from build123d import *

# Parameters (mm, degrees)
SKETCH1_W                                           = 52
SKETCH1_H                                           = 100
BOSS_EXTRUDE1_DEPTH                                 = 5
BOSS_EXTRUDE3_DEPTH                                 = 2.5
SKETCH7_R                                           = 2.25
BOSS_EXTRUDE4_DEPTH                                 = 2.5
FILLET2_R                                           = 0.25
SKETCH9_W                                           = 52
SKETCH9_H                                           = 2
BOSS_EXTRUDE5_DEPTH                                 = 50
BOSS_EXTRUDE7_DEPTH                                 = 52
CUT_EXTRUDE3_DEPTH                                  = 52
CUT_EXTRUDE4_DEPTH                                  = 2.5
BOSS_EXTRUDE8_DEPTH                                 = 52
BOSS_EXTRUDE9_DEPTH                                 = 4
LPATTERN1_COUNT                                     = 2
LPATTERN1_PITCH                                     = 48
SKETCH18_R                                          = 11.5
CUT_EXTRUDE5_DEPTH                                  = 2
CSK_FOR_M3_COUNTERSUNK_FLAT_HEAD_SCREW1_D           = 3.4
CSK_FOR_M3_COUNTERSUNK_FLAT_HEAD_SCREW1_DEPTH       = 5
CSK_FOR_M3_COUNTERSUNK_FLAT_HEAD_SCREW1_CSINK_D     = 6.3
CSK_FOR_M3_COUNTERSUNK_FLAT_HEAD_SCREW1_CSINK_ANGLE = 90
CSK_FOR_M3_COUNTERSUNK_FLAT_HEAD_SCREW1_TIP         = 1.021463052
BOSS_EXTRUDE10_DEPTH                                = 5
SKETCH23_R                                          = 1.75
CUT_EXTRUDE6_DEPTH                                  = 5
SKETCH24_W                                          = 6.6
SKETCH24_H                                          = 5.6
CUT_EXTRUDE7_DEPTH                                  = 2.5
SKETCH25_W                                          = 75
SKETCH25_H                                          = 5
SKETCH25_W_2                                        = 28.673992526
SKETCH25_H_2                                        = 8.232083525
CUT_EXTRUDE8_DEPTH                                  = 88


with BuildPart() as part:
    # Sketch1 → Boss-Extrude1 (new body)
    with BuildSketch(Plane(origin=(0, 0, 0), x_dir=(1, 0, 0), z_dir=(0, 1, 0))):
        Rectangle(SKETCH1_W, SKETCH1_H)
    extrude(amount=BOSS_EXTRUDE1_DEPTH)

    # Sketch2 → Boss-Extrude3 (add)
    with BuildSketch(Plane(origin=(0, 5, 0), x_dir=(1, 0, 0), z_dir=(0, 1, 0))):
        with BuildLine():
            Line((-26, 50), (26, 50))
            Line((26, 50), (26, 30))
            ThreePointArc((26, 30), (0, 22.708313008), (-26, 30))
            Line((-26, 30), (-26, 50))
        make_face()
    extrude(amount=BOSS_EXTRUDE3_DEPTH)

    # Sketch7 → Boss-Extrude4 (add)
    with BuildSketch(Plane(origin=(0, 7.5, 0), x_dir=(1, 0, 0), z_dir=(0, 1, 0))):
        with Locations((-7.5, 40.5)):
            Circle(SKETCH7_R)
        with Locations((7.5, 40.5)):
            Circle(SKETCH7_R)
    extrude(amount=BOSS_EXTRUDE4_DEPTH)

    # Fillet2
    fillet2_edges = [part.edges().sort_by_distance(p)[0] for p in [
        (-9.75, 10, -40.5),
        (5.25, 10, -40.5),
    ]]
    fillet(fillet2_edges, radius=FILLET2_R)

    # Sketch9 → Boss-Extrude5 (add)
    with BuildSketch(Plane(origin=(0, 5, 0), x_dir=(1, 0, 0), z_dir=(0, 1, 0))):
        with Locations((0, -3)):
            Rectangle(SKETCH9_W, SKETCH9_H)
    extrude(amount=BOSS_EXTRUDE5_DEPTH)

    # Sketch10 → Boss-Extrude7 (add)
    with BuildSketch(Plane.ZY.offset(26)):
        Polygon((4, 25), (25.126220325, 64.732641679), (23.36032514, 65.671584804), (4, 29.260108936), align=None)
    extrude(amount=-BOSS_EXTRUDE7_DEPTH)

    # Sketch11 → Cut-Extrude3 (cut)
    with BuildSketch(Plane.ZY.offset(26)):
        Polygon((4, 29.260108936), (2, 25.498656006), (2, 55), (4, 55), align=None)
    extrude(amount=-CUT_EXTRUDE3_DEPTH, mode=Mode.SUBTRACT)

    # Sketch13 → Cut-Extrude4 (cut)
    with BuildSketch(Plane(origin=(0, 7.5, 0), x_dir=(1, 0, 0), z_dir=(0, 1, 0))):
        with BuildLine():
            Line((-14.75, 24.933450371), (-14.75, 50))
            Line((-14.75, 50), (-26, 50))
            Line((-26, 50), (-26, 30))
            ThreePointArc((-26, 30), (-20.531880242, 27.118381074), (-14.75, 24.933450371))
        make_face()
        with BuildLine():
            Line((26, 50), (14.75, 50))
            Line((14.75, 50), (14.75, 24.933450371))
            ThreePointArc((14.75, 24.933450371), (20.531880242, 27.118381074), (26, 30))
            Line((26, 30), (26, 50))
        make_face()
    extrude(amount=-CUT_EXTRUDE4_DEPTH, mode=Mode.SUBTRACT)

    # Sketch16 → Boss-Extrude8 (add)
    with BuildSketch(Plane.ZY.offset(26)):
        Polygon((4.469471563, 25.882947593), (43.744583775, 5), (39.744583775, 5), (4, 24.005732324), (4, 25), align=None)
    extrude(amount=-BOSS_EXTRUDE8_DEPTH)

    # Sketch17 → Boss-Extrude9 (add)
    with BuildSketch(Plane.ZY.offset(26)):
        Polygon((25.126220325, 64.732641679), (25.126220325, 5), (21.872291888, 5), (21.872291888, 58.612892349), align=None)
    boss_extrude9 = extrude(amount=-BOSS_EXTRUDE9_DEPTH)

    # LPattern1: Boss-Extrude9 ×2
    with Locations(*[(i * LPATTERN1_PITCH, 0, 0) for i in range(1, LPATTERN1_COUNT)]):
        add(boss_extrude9)

    # Sketch18 → Cut-Extrude5 (cut)
    with BuildSketch(Plane(origin=(0, 4.790956687, -9.010479036), x_dir=(-1, 0, 0), z_dir=(0, 0.469471563, -0.882947593))):
        with Locations((0, 45.951576073)):
            Circle(SKETCH18_R)
    extrude(amount=-CUT_EXTRUDE5_DEPTH, mode=Mode.SUBTRACT)

    # CSK for M3 Countersunk Flat Head Screw1
    with Locations(Plane(origin=(0, 4.790956687, -9.010479036), x_dir=(-1, 0, 0), z_dir=(0, 0.469471563, -0.882947593))):
        with Locations((-15.5, 61.45224807), (15.5, 61.45224807), (15.5, 30.45224807), (-15.5, 30.45224807)):
            CounterSinkHole(CSK_FOR_M3_COUNTERSUNK_FLAT_HEAD_SCREW1_D / 2, CSK_FOR_M3_COUNTERSUNK_FLAT_HEAD_SCREW1_CSINK_D / 2, depth=CSK_FOR_M3_COUNTERSUNK_FLAT_HEAD_SCREW1_DEPTH, counter_sink_angle=CSK_FOR_M3_COUNTERSUNK_FLAT_HEAD_SCREW1_CSINK_ANGLE)
            with Locations((0, 0, -(CSK_FOR_M3_COUNTERSUNK_FLAT_HEAD_SCREW1_DEPTH + CSK_FOR_M3_COUNTERSUNK_FLAT_HEAD_SCREW1_TIP / 2))):  # 118° drill point
                Cone(0, CSK_FOR_M3_COUNTERSUNK_FLAT_HEAD_SCREW1_D / 2, CSK_FOR_M3_COUNTERSUNK_FLAT_HEAD_SCREW1_TIP, mode=Mode.SUBTRACT)

    # Sketch22 → Boss-Extrude10 (add)
    with BuildSketch(Plane.XZ):
        Polygon((26, 75), (-61, 75), (-61, 0), (-26, 0), (-26, 50), (26, 50), align=None)
    extrude(amount=-BOSS_EXTRUDE10_DEPTH)

    # Sketch23 → Cut-Extrude6 (cut)
    with BuildSketch(Plane(origin=(0, 5, 0), x_dir=(1, 0, 0), z_dir=(0, 1, 0))):
        with Locations((-31.5, -5.5)):
            Circle(SKETCH23_R)
        with Locations((-55.5, -5.5)):
            Circle(SKETCH23_R)
        with Locations((-55.5, -69.5)):
            Circle(SKETCH23_R)
        with Locations((-31.5, -69.5)):
            Circle(SKETCH23_R)
    extrude(amount=-CUT_EXTRUDE6_DEPTH, mode=Mode.SUBTRACT)

    # Sketch24 → Cut-Extrude7 (cut)
    with BuildSketch(Plane.XZ):
        with Locations((-31.5, 69.5)):
            Rectangle(SKETCH24_W, SKETCH24_H)
        with Locations((-55.5, 69.5)):
            Rectangle(SKETCH24_W, SKETCH24_H)
        with Locations((-31.5, 5.5)):
            Rectangle(SKETCH24_W, SKETCH24_H)
        with Locations((-55.5, 5.5)):
            Rectangle(SKETCH24_W, SKETCH24_H)
    extrude(amount=-CUT_EXTRUDE7_DEPTH, mode=Mode.SUBTRACT)

    # Sketch25 → Cut-Extrude8 (cut, through all)
    with BuildSketch(Plane.ZY.offset(61)):
        Polygon((0, 0), (0, 5), (-21.326007474, 5), (-50, 5), (-50, 0), align=None)
        with Locations((37.5, 2.5)):
            Rectangle(SKETCH25_W, SKETCH25_H)
        with Locations((-35.663003737, 9.116041763)):
            Rectangle(SKETCH25_W_2, SKETCH25_H_2)
    extrude(amount=-CUT_EXTRUDE8_DEPTH, mode=Mode.SUBTRACT)


solid = part.part
Check sheet for the modelled part. Datum: model origin and axes. Units: mm. A direction names the side the tool comes from. Round coordinates to 2 decimals unless told otherwise and drop trailing zeros. Order: outer loops, then holes, each group sorted by start corner. A loop starts at its lowest first (then second) coordinate and runs counter-clockwise, first axis right, second up.
Q1. Cross-section at B-B, the plane x = -23. Enter the section's corners in (y, z).
Filled sheet:
outline: (5, 2) - (25.5, 2) - (65.67, 23.36) - (64.73, 25.13) - (14.9, 25.13) - (5, 43.74) - (5, 39.74) - (12.77, 25.13) - (5, 25.13) - (5, 21.87) - (14.5, 21.87) - (24.01, 4) - (5, 4) - close; hole (16.63, 21.87) - (25.88, 4.47) - (58.61, 21.87) - close
Q2. Draft check along X on faces 1 (the face through (-26, 31, 23)), 2 (the face through (-13.88, 31.32, 7.05)), 3 (the face through (24, 5, 24)), 4 (the face through (26, 28, 23)). Enter one of: pulls with the +X half, pulls with the -X half, needs draft (parallel to the pull), parting line crosses it, or undercut.
Filled sheet:
face 1: pulls with the -X half
face 2: undercut
face 3: needs draft
face 4: pulls with the +X half
Q3. Set-up check for faces 5 (the face through (24, 10, 21.872)), 6 (the face through (0, 5, 42)), 7 (the face through (-24, 37, 21.872)), 8 (the face through (22, 10, 24)): record each of +Z, -Z, +X, -X, +Y, -Y from which the full face is reachable in a straight line by a thin tool's end or side.
Filled sheet:
face 5: +X, -X, -Y
face 6: +Z, -Z, +X, -X, -Y
face 7: +X, -X
face 8: -Y
Q4. Scan lines: L1, parallel to X at y = 58, z = 24.5; L2, parallel to Z at x = 2.5, y = 12.5; L3, parallel to Z at x = -19.5, y = 13.5. Record each from-to range of solid material in increasing order.
Filled sheet:
L1: x = -26 to -22, 22 to 26
L2: z = 2 to 4, 25.64 to 29.64
L3: z = 2 to 4, 23.76 to 27.76
Q5. Cross-section at C-C, the plane z = 17. Give the number of separate pieces and of enclosed holes in the cut face, plus the area to 3 significant figures.
Filled sheet:
separate pieces: 3
enclosed holes: 0
area: 259 mm2
Q6. Cross-section at A-A, the plane x = 10. Enter the section's corners in (y, z).
Filled sheet:
outline: (5, 2) - (25.5, 2) - (40.35, 9.9) - (39.41, 11.66) - (25.88, 4.47) - (5, 43.74) - (5, 39.74) - (24.01, 4) - (5, 4) - close; (49.44, 16.99) - (50.38, 15.23) - (65.67, 23.36) - (64.73, 25.13) - close
Q7. Depth check by flat-ended pin: P1, Ø4, axis at x = -5, y = 15.5, coming from the +Z side; P2, Ø12, axis at x = 7.5, y = 46, coming from the -Z side; P3, Ø4.5, axis at x = 23, y = 7, coming from the +Z side. Enter the tip coordinate at first touch or a pass-through.
Filled sheet:
P1: stops at z = 27.76
P2: stops at z = 10.04
P3: stops at z = 43.74
